from build123d import *

# Parameters (mm, degrees)
BOSS_EXTRUDE1_DEPTH = 50
SKETCH3_W           = 8
SKETCH3_H           = 10
CUT_EXTRUDE5_DEPTH  = 18


with BuildPart() as part:
    # Sketch2 → Boss-Extrude1 (new body)
    with BuildSketch(Plane(origin=(0, 0, 0), x_dir=(1, 0, 0), z_dir=(0, 1, 0))):
        with BuildLine():
            ThreePointArc((-23.68807717, -23.68807717), (-33.5, 0), (-23.68807717, 23.68807717))
            Line((-23.68807717, 23.68807717), (-29.68807717, 23.68807717))
            add(Edge.make_bspline(
                [(-29.68807717, 23.68807717), (-47.221735333, 1.183613852), (-33.68807717, -23.68807717)],
                knots=[0, 0, 0, 1, 1, 1], degree=2))
            Line((-33.68807717, -23.68807717), (-23.68807717, -23.68807717))
        make_face()
    extrude(amount=BOSS_EXTRUDE1_DEPTH)

    # Sketch3 → Cut-Extrude5 (cut)
    with BuildSketch(Plane.XY.offset(23.68807717)):
        with Locations((-37.68807717, 12.5)):
            Rectangle(SKETCH3_W, SKETCH3_H)
    extrude(amount=-CUT_EXTRUDE5_DEPTH, mode=Mode.SUBTRACT)


solid = part.part
The listing builds one solid part. Answer for the finished solid, in the listing's coordinates (mm). A direction names the side the tool comes from. Coordinates: 2 decimals unless noted, no trailing zeros. Write each loop counter-clockwise with the first axis right and the second up, starting at its lowest first coordinate (ties: lowest second). Pieces come first, ordered by that corner, then holes. Notation, with made-up numbers: M 49,72 L 94,72 A14 ccw 94,97 Z; hole C 84,35.5 d4. An arc over 180 degrees is marked long. Write each question's results on one line, items separated by ' | '.
Item 1: Given P1, Ø1.5, axis at y = 39, z = 12, coming from the +X side; P2, Ø2, axis at y = 17.5, z = 3.5, coming from the +X side; P3, Ø1.5, axis at y = 27, z = 16, coming from the -X side, each flat-ended and moving along its own axis, determine where each tip first touches the part or whether it passes through.
Answer below:
P1: x = -30.98 | P2: x = -33.2 | P3: x = -37.41
Item 2: The part is cut by section B-B on x = -26.5. Determine the outline of the cut face in (y, z), and give its area (3 significant figures).
Answer below:
outline: M 0,-23.69 L 50,-23.69 L 50,-20.49 L 0,-20.49 Z; M 0,20.49 L 50,20.49 L 50,23.69 L 0,23.69 Z | area: 319 mm2
Item 3: Which of the six approach directions +Z, -Z, +X, -X, +Y, -Y give full straight-line access (tool end or side, diameter ignored) to faces 1 (the face through (-34, 50, 2)), 2 (the face through (-36, 7.5, 13))?
Answer below:
face 1: +Z, -Z, +X, -X, +Y | face 2: +Z, -X
Item 4: For a pull along Y with two mould halves and no side action, classify faces 3 (the face through (-29, 25, 23.688)), 4 (the face through (-36, 17.5, 13)), 5 (the face through (-34, 0, 2)) as released by +Y, released by -Y, zero draft, split by the parting line, or undercut.
Answer below:
face 3: zero draft | face 4: undercut | face 5: released by -Y
Item 5: The part is cut by section A-A on x = -29. Determine the outline of the cut face in (y, z), and give its area (3 significant figures).
Answer below:
outline: M 0,-23.69 L 50,-23.69 L 50,-16.77 L 0,-16.77 Z; M 0,16.77 L 50,16.77 L 50,23.69 L 0,23.69 Z | area: 692 mm2
Item 6: Consider probe 1 along Y at (x, z) = (-36.5, 16); probe 2 along Z at (x, y) = (-29.25, 33); probe 3 along Z at (x, y) = (-29.5, 6). Determine where each line is inside the solid, lowest interval first. Write a range as [from, to].
Answer below:
probe 1: [0, 7.5], [17.5, 50] | probe 2: [-23.69, -16.33], [16.33, 23.69] | probe 3: [-23.69, -15.87], [15.87, 23.69]
